Autodesk Inventor part; units mm, degrees
ref_plane "YZ Plane" through (0, 0, 0) normal (1, 0, 0) x (0, 1, 0)
ref_plane "XZ Plane" through (0, 0, 0) normal (0, 1, 0) x (-1, 0, 0)
ref_plane "XY Plane" through (0, 0, 0) normal (0, 0, 1) x (1, 0, 0)
sketch "Skizze1" plane through (0, 0, 0) normal (0, 1, 0) x (-1, 0, 0)
  line L0 (0, 0) -> (-130, 0)
  line L1 (-140, -10) -> (-140, -90)
  line L2 (-130, -100) -> (0, -100)
  line L3 (10, -10) -> (10, -90)
  arc A0 (0, -100) -> (10, -90) centre (0, -90) ccw
  arc A1 (-140, -90) -> (-130, -100) centre (-130, -90) ccw
  arc A2 (-130, 0) -> (-140, -10) centre (-130, -10) ccw
  arc A3 (10, -10) -> (0, 0) centre (0, -10) ccw
  dimension "d0" = 150
  dimension "d1" = 100
  dimension "d2" = 10
extrude "Extrusion1" add sketch "Skizze1" along normal blind 2
sketch "Skizze2" plane through (0, 2, 0) normal (0, 1, 0) x (1, 0, 0)
  line L0 (0, 0) -> (130, 0)
  arc A0 (130, 0) -> (140, 10) centre (130, 10) ccw
  line L1 (140, 10) -> (140, 90)
  arc A1 (140, 90) -> (130, 100) centre (130, 90) ccw
  line L2 (130, 100) -> (0, 100)
  arc A2 (0, 100) -> (-10, 90) centre (0, 90) ccw
  line L3 (-10, 90) -> (-10, 10)
  arc A3 (-10, 10) -> (0, 0) centre (0, 10) ccw
  line L4 (0, 2) -> (130, 2)
  line L5 (130, 2) -> (130, 5.5)
  line L6 (130, 5.5) -> (0, 5.5)
  line L7 (0, 5.5) -> (0, 2)
  line L8 (138, 10) -> (134.5, 10)
  line L9 (134.5, 10) -> (134.5, 90)
  line L10 (134.5, 90) -> (138, 90)
  line L11 (138, 90) -> (138, 10)
  line L12 (130, 98) -> (0, 98)
  line L13 (0, 98) -> (0, 94.5)
  line L14 (0, 94.5) -> (130, 94.5)
  line L15 (130, 94.5) -> (130, 98)
  line L16 (-8, 90) -> (-4.5, 90)
  line L17 (-4.5, 90) -> (-4.5, 10)
  line L18 (-4.5, 10) -> (-8, 10)
  line L19 (-8, 10) -> (-8, 90)
  line L20 (65, 2) -> (65, 0) construction
  line L21 (0, 0) -> (130, 0) construction
  line L22 (138, 50) -> (140, 50) construction
  line L23 (140, 10) -> (140, 90) construction
  line L24 (65, 98) -> (65, 100) construction
  line L25 (130, 100) -> (0, 100) construction
  line L26 (-8, 50) -> (-10, 50) construction
  line L27 (-10, 90) -> (-10, 10) construction
  line L28 (140, 88) -> (138, 88)
  line L29 (134.5, 88) -> (132.5, 88)
  line L30 (132.5, 88) -> (132.5, 92.5)
  line L31 (132.5, 92.5) -> (128, 92.5)
  line L32 (128, 92.5) -> (128, 94.5)
  line L33 (128, 98) -> (128, 100)
  line L34 (140, 12) -> (138, 12)
  line L35 (134.5, 12) -> (132.5, 12)
  line L36 (132.5, 12) -> (132.5, 7.5)
  line L37 (132.5, 7.5) -> (128, 7.5)
  line L38 (128, 7.5) -> (128, 5.5)
  line L39 (128, 2) -> (128, 0)
  line L40 (2, 0) -> (2, 2)
  line L41 (2, 5.5) -> (2, 7.5)
  line L42 (2, 7.5) -> (-2.5, 7.5)
  line L43 (-2.5, 7.5) -> (-2.5, 12)
  line L44 (-2.5, 12) -> (-4.5, 12)
  line L45 (-8, 12) -> (-10, 12)
  line L46 (-10, 88) -> (-8, 88)
  line L47 (-4.5, 88) -> (-2.5, 88)
  line L48 (-2.5, 88) -> (-2.5, 92.5)
  line L49 (-2.5, 92.5) -> (2, 92.5)
  line L50 (2, 92.5) -> (2, 94.5)
  line L51 (2, 98) -> (2, 100)
  line L52 (-2, 92) -> (132, 92)
  line L53 (132, 92) -> (132, 8)
  line L54 (132, 8) -> (-2, 8)
  line L55 (-2, 8) -> (-2, 92)
  line L56 (130, 90) -> (0, 90)
  line L57 (0, 90) -> (0, 10)
  line L58 (0, 10) -> (130, 10)
  line L59 (130, 10) -> (130, 90)
  line L60 (-2.5, 92.5) -> (0, 90) construction
  line L61 (132.5, 92.5) -> (130, 90) construction
  line L62 (132.5, 7.5) -> (130, 10) construction
  line L63 (-2.5, 7.5) -> (0, 10) construction
  line L64 (2, 88) -> (128, 88)
  line L65 (128, 88) -> (128, 12)
  line L66 (128, 12) -> (2, 12)
  line L67 (2, 12) -> (2, 88)
  line L68 (132.5, 12) -> (132, 12)
  line L69 (128, 7.5) -> (128, 8)
  line L70 (132.5, 88) -> (132, 88)
  line L71 (128, 92.5) -> (128, 92)
  line L72 (2, 92.5) -> (2, 92)
  line L73 (-2.5, 88) -> (-2, 88)
  line L74 (2, 7.5) -> (2, 8)
  line L75 (-2.5, 12) -> (-2, 12)
  point P0 (130, 3.75)
  point P1 (128, 0)
  dimension "d5" = 3.5
  dimension "d6" = 2
  dimension "d7" = 2
  dimension "d12" = 2
  dimension "d13" = 2
  dimension "d14" = 0.5
  dimension "d15" = 2
extrude "Extrusion2" add sketch "Skizze2" along normal blind 2 contours A3 L3 L45 L19 L18 L17 L44 L43 L42 L41 L6 L7 L4 L40 L0 | L40 L4 L39 L0 | L39 L4 L5 L6 L38 L37 L36 L35 L9 L8 L11 L34 L1 A0 L0 | L3 L46 L19 L45 | L3 A2 L2 L51 L12 L13 L14 L50 L49 L48 L47 L17 L16 L19 L46 | L34 L11 L28 L1 | L28 L11 L10 L9 L29 L30 L31 L32 L14 L15 L12 L33 L2 A1 L1 | L2 L33 L12 L51
extrude "Extrusion4" add sketch "Skizze2" along normal blind 20 contours L41 L74 L54 L69 L38 L6 | L42 L43 L75 L55 L54 L74 | L17 L47 L73 L55 L75 L44 | L69 L54 L53 L68 L36 L37 | L48 L49 L72 L52 L55 L73 | L35 L68 L53 L70 L29 L9 | L14 L32 L71 L52 L72 L50 | L70 L53 L52 L71 L31 L30 | L59 L58 L57 L56
sketch "Skizze3" plane through (0, 22, 0) normal (0, 1, 0) x (1, 0, 0)
  line L0 (132.5, 7.5) -> (132.5, 12)
  line L1 (132.5, 12) -> (134.5, 12)
  line L2 (134.5, 12) -> (134.5, 88)
  line L3 (134.5, 88) -> (132.5, 88)
  line L4 (132.5, 88) -> (132.5, 92.5)
  line L5 (132.5, 92.5) -> (128, 92.5)
  line L6 (128, 92.5) -> (128, 94.5)
  line L7 (128, 94.5) -> (2, 94.5)
  line L8 (2, 94.5) -> (2, 92.5)
  line L9 (2, 92.5) -> (-2.5, 92.5)
  line L10 (-2.5, 92.5) -> (-2.5, 88)
  line L11 (-2.5, 88) -> (-4.5, 88)
  line L12 (-4.5, 88) -> (-4.5, 12)
  line L13 (-4.5, 12) -> (-2.5, 12)
  line L14 (-2.5, 12) -> (-2.5, 7.5)
  line L15 (-2.5, 7.5) -> (2, 7.5)
  line L16 (2, 7.5) -> (2, 5.5)
  line L17 (2, 5.5) -> (128, 5.5)
  line L18 (128, 5.5) -> (128, 7.5)
  line L19 (128, 7.5) -> (132.5, 7.5)
  line L20 (132, 8) -> (-2, 8)
  line L21 (-2, 8) -> (-2, 92)
  line L22 (-2, 92) -> (132, 92)
  line L23 (132, 92) -> (132, 8)
  line L24 (132, 12.5) -> (132, 8)
  line L25 (132, 8) -> (127.5, 8)
  line L26 (127.5, 8) -> (127.5, 6)
  line L27 (127.5, 6) -> (2.5, 6)
  line L28 (2.5, 6) -> (2.5, 8)
  line L29 (2.5, 8) -> (-2, 8)
  line L30 (-2, 8) -> (-2, 12.5)
  line L31 (-2, 12.5) -> (-4, 12.5)
  line L32 (-4, 12.5) -> (-4, 87.5)
  line L33 (-4, 87.5) -> (-2, 87.5)
  line L34 (-2, 87.5) -> (-2, 92)
  line L35 (-2, 92) -> (2.5, 92)
  line L36 (2.5, 92) -> (2.5, 94)
  line L37 (2.5, 94) -> (127.5, 94)
  line L38 (127.5, 94) -> (127.5, 92)
  line L39 (127.5, 92) -> (132, 92)
  line L40 (132, 92) -> (132, 87.5)
  line L41 (132, 87.5) -> (134, 87.5)
  line L42 (134, 87.5) -> (134, 12.5)
  line L43 (134, 12.5) -> (132, 12.5)
  line L44 (2.5, 6) -> (2.5, 5.5)
  line L45 (-4, 12.5) -> (-4.5, 12.5)
  line L46 (-4.5, 10) -> (-4.5, 90)
  line L47 (-4, 87.5) -> (-4.5, 87.5)
  line L48 (2.5, 94) -> (2.5, 94.5)
  line L49 (0, 94.5) -> (130, 94.5)
  line L50 (127.5, 94) -> (127.5, 94.5)
  line L51 (134, 87.5) -> (134.5, 87.5)
  line L52 (134, 12.5) -> (134.5, 12.5)
  line L53 (127.5, 6) -> (127.5, 5.5)
  line L54 (2, 5.5) -> (128, 5.5)
  point P0 (0, 0)
  dimension "d22" = 0.5
extrude "Extrusion5" cut sketch "Skizze3" against normal up to surface (18 mm away) contours L19 L18 L17 L53 L26 L20 L23 L43 L52 L2 L1 L0 | L51 L41 L23 L22 L38 L50 L7 L6 L5 L4 L3 L2 | L17 L16 L15 L14 L13 L12 L45 L31 L21 L20 L28 L44 | L22 L21 L33 L47 L12 L11 L10 L9 L8 L7 L48 L36
sketch "Skizze4" plane through (0, 2, 0) normal (0, 1, 0) x (1, 0, 0)
  line L0 (2, 88) -> (2, 12)
  line L1 (2, 12) -> (128, 12)
  line L2 (128, 12) -> (128, 88)
  line L3 (128, 88) -> (2, 88)
  line L4 (128, 88) -> (2, 88)
  line L5 (128, 12) -> (2, 12)
  line L6 (12, 88) -> (118, 88)
  line L7 (118, 88) -> (118, 12)
  line L8 (118, 12) -> (12, 12)
  line L9 (12, 12) -> (12, 88)
  line L10 (2, 88) -> (128, 88)
  point P0 (0, 0)
  point P1 (65, 88)
  point P2 (12, 12)
  point P3 (118, 12)
  point P4 (118, 88)
  dimension "d25" = 10
extrude "Extrusion6" cut sketch "Skizze4" against normal through all contours L3 L7 L1 L9
sketch "Skizze6" plane through (130, 2, -94.5) normal (0, 0, -1) x (-1, 0, 0)
  line L0 (130, 2) -> (127.5, 2)
  line L1 (127.5, 2) -> (127.5, 20)
  line L2 (2.5, 20) -> (127.5, 20)
  line L3 (2.5, 20) -> (2.5, 2)
  line L4 (0, 2) -> (2.5, 2)
  line L5 (0, 0) -> (0, 2)
  line L6 (130, 0) -> (0, 0)
  line L7 (130, 0) -> (130, 2)
  line L8 (128, 20) -> (2, 20)
  line L9 (55, 20) -> (75, 20)
  line L10 (75, 20) -> (75, 0)
  line L11 (75, 0) -> (55, 0)
  line L12 (55, 0) -> (55, 20)
  point P0 (130, -2)
  point P1 (65, 20)
  point P2 (55, 20)
  point P3 (55, 0)
  point P4 (75, 20)
  dimension "d31" = 20
extrude "Extrusion8" cut sketch "Skizze6" against normal up to surface (6.5 mm away) contours L6 L12 L2 L10
sketch "Skizze7" plane through (0, 0, 0) normal (0, -1, 0) x (1, 0, 0)
  line L0 (118, -12) -> (118, -88)
  line L1 (118, -88) -> (12, -88)
  line L2 (12, -88) -> (12, -12)
  line L3 (12, -12) -> (118, -12)
  line L4 (0, 0) -> (130, 0)
  arc A0 (0, 0) -> (-10, -10) centre (0, -10) ccw
  line L5 (-10, -90) -> (-10, -10)
  arc A1 (-10, -90) -> (0, -100) centre (0, -90) ccw
  line L6 (130, -100) -> (0, -100)
  arc A2 (130, -100) -> (140, -90) centre (130, -90) ccw
  line L7 (140, -10) -> (140, -90)
  arc A3 (140, -10) -> (130, 0) centre (130, -10) ccw
  line L8 (118, -88) -> (12, -88)
  line L9 (68.5, -88) -> (61.5, -88)
  line L10 (61.5, -88) -> (61.5, -82)
  line L11 (61.5, -82) -> (68.5, -82)
  line L12 (68.5, -82) -> (68.5, -88)
  line L13 (61.5, -82) -> (63.5, -82)
  line L14 (63.5, -82) -> (63.5, -84)
  line L15 (63.5, -84) -> (61.5, -84)
  line L16 (61.5, -84) -> (61.5, -82)
  line L17 (68.5, -82) -> (66.5, -82)
  line L18 (66.5, -82) -> (66.5, -84)
  line L19 (66.5, -84) -> (68.5, -84)
  line L20 (68.5, -84) -> (68.5, -82)
  point P0 (65, -88)
  point P1 (61.5, -84)
  dimension "d39" = 6
  dimension "d40" = 7
  dimension "d41" = 2
extrude "Extrusion9" add sketch "Skizze7" against normal up to surface (22 mm away) contours L19 L18 L11 L12 | L10 L11 L14 L15
extrude "Extrusion10" add sketch "Skizze7" against normal blind 2 contours L1 L10 L15 L14 L11 L18 L19 L12
properties part number "bottom"
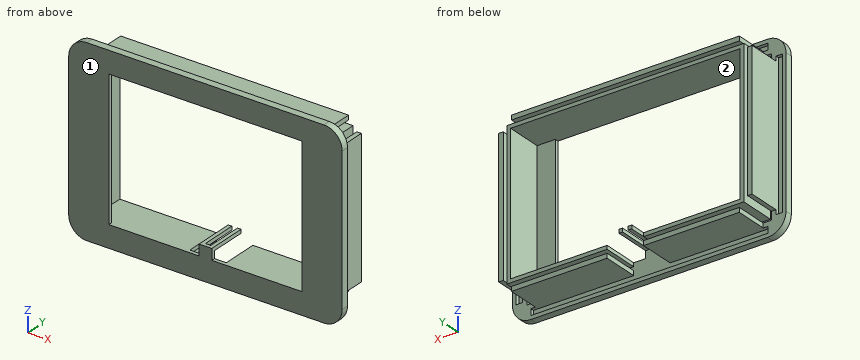
Geometry: final body of the model. Coordinates: model frame, mm. Face numbers are marked on the shaded views. Give positions to 0.01 mm unless a question says otherwise; leave off trailing zeros. Loops run counter-clockwise (first coordinate to the right, second up) from the corner with the lowest first, then second, coordinate; pieces in that order, holes last. Notation, with made-up numbers: (-31, 23) -> (6, 23) arc R21 cw to (6, 34) -> close; hole circle Ø4 at (34, 69.5). An arc over 180 degrees is marked (long way). Put each result on its own line as item: value.
1. Cut plane A-A (z = -73). Return the cut outline in (x, y).
Taken from the geometry:
outline: (-10, 0) -> (12, 0) -> (12, 2) -> (2, 2) -> (2, 22) -> (0, 22) -> (0, 2) -> (-2, 2) -> (-2, 22) -> (-4.5, 22) -> (-4.5, 2) -> (-8, 2) -> (-8, 4) -> (-10, 4) -> close; (118, 0) -> (140, 0) -> (140, 4) -> (138, 4) -> (138, 2) -> (134.5, 2) -> (134.5, 22) -> (132, 22) -> (132, 2) -> (130, 2) -> (130, 22) -> (128, 22) -> (128, 2) -> (118, 2) -> close
2. Pull-direction query (X, two-part tool) for the marked faces 1 and 2; classes: released by +X, released by -X, zero draft, split by the parting line, or undercut.
Taken from the geometry:
face 1: zero draft
face 2: undercut
3. Pin query (flat end, axial travel): P1, Ø8, axis at x = 83, y = 13, coming from the +Z side; P2, Ø2, axis at y = 3, z = -96.5, coming from the +X side; P3, Ø5, axis at x = 49.5, y = 15.5, coming from the -Z side. Return the tip coordinate at first contact, or that it passes through.
Taken from the geometry:
P1: stops at z = -5.5
P2: stops at x = 138.35
P3: stops at z = -94.5
4. Cut plane B-B (x = 19). Return the cut outline in (y, z).
Taken from the geometry:
outline: (0, -100) -> (4, -100) -> (4, -98) -> (2, -98) -> (2, -94.5) -> (22, -94.5) -> (22, -92) -> (2, -92) -> (2, -90) -> (22, -90) -> (22, -88) -> (0, -88) -> close; (0, -12) -> (22, -12) -> (22, -10) -> (2, -10) -> (2, -8) -> (22, -8) -> (22, -5.5) -> (2, -5.5) -> (2, -2) -> (4, -2) -> (4, 0) -> (0, 0) -> close
5. Cut plane D-D (x = 58). Return the cut outline in (y, z), plus the area to 3 significant figures.
Taken from the geometry:
outline: (0, -100) -> (4, -100) -> (4, -98) -> (2, -98) -> (2, -88) -> (0, -88) -> close; (0, -12) -> (22, -12) -> (22, -10) -> (2, -10) -> (2, -8) -> (22, -8) -> (22, -5.5) -> (2, -5.5) -> (2, -2) -> (4, -2) -> (4, 0) -> (0, 0) -> close
area: 146 mm2
6. Cut plane C-C (y = 8.75). Count the separate pieces of the cut face and the enclosed holes in it, plus the area to 3 significant figures.
Taken from the geometry:
separate pieces: 8
enclosed holes: 0
area: 1,740 mm2
7. Ray query, line 1 along X through (y, z) = (6, -51.5); line 2 along Z through (x, y) = (53.5, 19.5); line 3 along Z through (x, y) = (69.5, 8.75). Return the intervals inside material, ascending. Write a range as [from, to].
Taken from the geometry:
line 1: x = [-4.5, -2], [0, 2], [128, 130], [132, 134.5]
line 2: z = [-94.5, -92], [-90, -88], [-12, -10], [-8, -5.5]
line 3: z = [-12, -10], [-8, -5.5]
